Drawing for the job (mm, zero at the part's lowest x, y, z). A direction names the side the tool comes from. Coordinates: 2 decimals unless noted, no trailing zeros. Write each loop counter-clockwise with the first axis right and the second up, starting at its lowest first coordinate (ties: lowest second). Pieces come first, ordered by that corner, then holes. Notation, with made-up numbers: (85, 70) -> (95, 70) arc R12 ccw to (95, 74) -> close; hole circle Ø6 at (-38.75, 13.5). An arc over 180 degrees is marked (long way). Write item = value, one per line. Start each with the question number.
Q1. Band-saw the part on C-C, the plane x = 5. List the corners of the cut face in (y, z).
Q2. Probe line 1 (X direction, y = 11, z = 8.5); line 2 (Y direction, x = 4, z = 4); line 3 (Z direction, x = 8.75, y = 3.75). List the from-to ranges inside material, lowest first.
Q3. Band-saw the part on A-A, the plane y = 6. List the corners of the cut face in (x, z).
Q4. Tool access for the marked faces 1 and 2: list every direction of +Z, -Z, +X, -X, +Y, -Y with a clear straight run to the whole face (end or side of a thin tool).
Q5. Pin check, flat tips, straight feed: P1, Ø5, axis at x = 16, y = 3.5, coming from the +Z side; P2, Ø5, axis at x = 17.5, y = 1.5, coming from the -Z side; P3, Ø1, axis at x = 6.5, z = 4.5, coming from the +Y side. Stop position of each tip, or through.
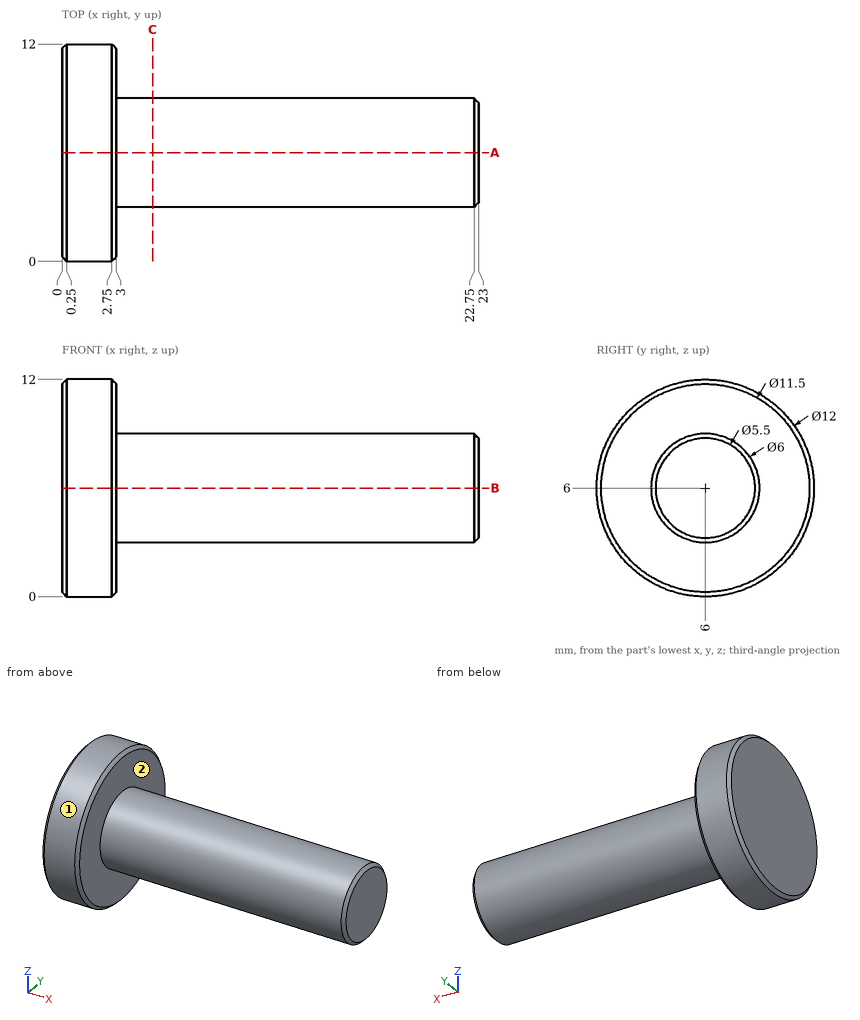
Ans:
q1.outline = circle Ø6 at (6, 6)
q2.line_1 = 0 to 3
q2.line_2 = 3.76 to 8.24
q2.line_3 = 4.02 to 7.98
q3.outline = (0, 0.25) -> (0.25, 0) -> (2.75, 0) -> (3, 0.25) -> (3, 3) -> (22.75, 3) -> (23, 3.25) -> (23, 8.75) -> (22.75, 9) -> (3, 9) -> (3, 11.75) -> (2.75, 12) -> (0.25, 12) -> (0, 11.75) -> close
q4.face_1 = +X, -X
q4.face_2 = +X
q5.P1 = 9
q5.P2 = 3.76
q5.P3 = 8.83
